Can you work these out from the drawing? Everything is in mm from the part's minimum corner. Give positions to 0.01 mm unless a question says otherwise; leave off trailing zeros. Loops run counter-clockwise (first coordinate to the right, second up) from the corner with the lowest first, then second, coordinate; pieces in that order, holes last. Notation, with made-up numbers: (22, -6.5) -> (81, -6.5) arc R19 ccw to (81, 15.5) -> close; hole circle Ø1 at (54, -25.5). An arc over 180 degrees is marked (long way). Write item = value, one per line. Start each with the question number.
1) I want a section at B-B (z = 0.65). Count the separate pieces of the cut face and the enclosed holes in it, and give its area (3 significant figures).
2) I want a section at C-C (x = 90). List the corners of the cut face in (y, z) for me, and give its area (3 significant figures).
3) I want a section at A-A (y = 15). List the corners of the cut face in (x, z) for me, and give its area (3 significant figures).
4) If we mould it in two halves opening along Z, with no side actions, what happens to the marked faces 1 and 2? For each: +Z half, -Z half, draft (parallel to the pull), parting line (faces both ways), or undercut.
5) I need wall thicknesses on probe 1 along Y at (x, z) = (90, 1.4); probe 2 along X at (y, z) = (6.5, 1.25); probe 3 along X at (y, z) = (34, 0.75). Which ranges of each line are inside material? Lowest first, please. Write a range as from..to.
6) I want a section at D-D (y = 45). List the corners of the cut face in (x, z) for me, and give its area (3 significant figures).
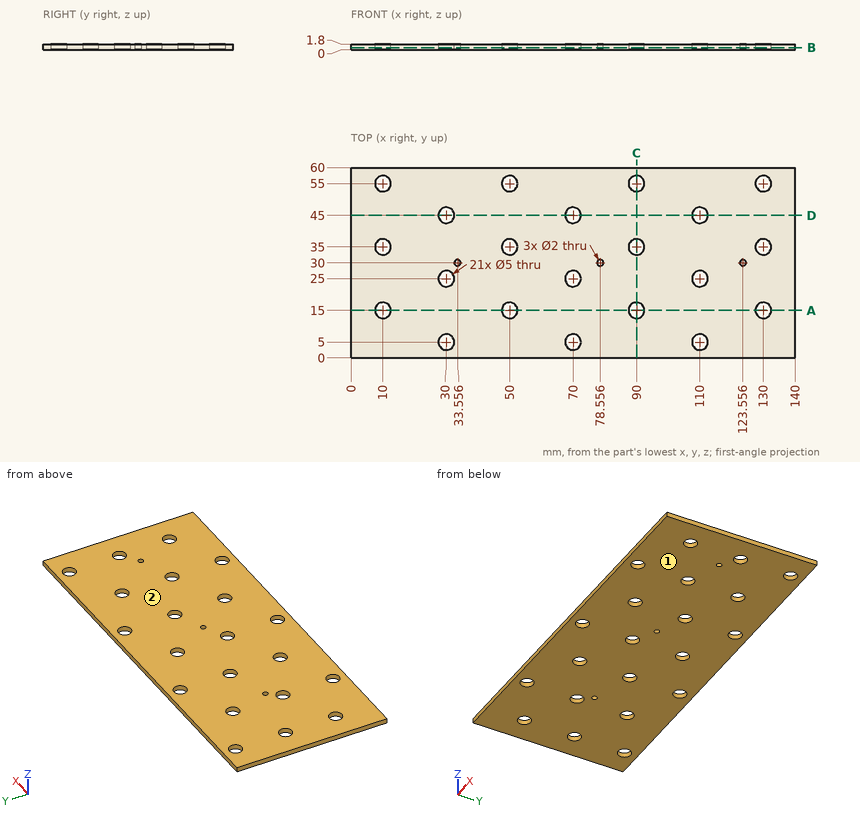
Answer list:
q1.separate_pieces = 1
q1.enclosed_holes = 24
q1.area = 7,980 mm^2
q2.outline = (0, 0) -> (12.5, 0) -> (12.5, 1.8) -> (0, 1.8) -> close; (17.5, 0) -> (32.5, 0) -> (32.5, 1.8) -> (17.5, 1.8) -> close; (37.5, 0) -> (52.5, 0) -> (52.5, 1.8) -> (37.5, 1.8) -> close; (57.5, 0) -> (60, 0) -> (60, 1.8) -> (57.5, 1.8) -> close
q2.area = 81.0 mm^2
q3.outline = (0, 0) -> (7.5, 0) -> (7.5, 1.8) -> (0, 1.8) -> close; (12.5, 0) -> (47.5, 0) -> (47.5, 1.8) -> (12.5, 1.8) -> close; (52.5, 0) -> (87.5, 0) -> (87.5, 1.8) -> (52.5, 1.8) -> close; (92.5, 0) -> (127.5, 0) -> (127.5, 1.8) -> (92.5, 1.8) -> close; (132.5, 0) -> (140, 0) -> (140, 1.8) -> (132.5, 1.8) -> close
q3.area = 216 mm^2
q4.face_1 = -Z half
q4.face_2 = +Z half
q5.probe_1 = 0..12.5, 17.5..32.5, 37.5..52.5, 57.5..60
q5.probe_2 = 0..28, 32..68, 72..108, 112..140
q5.probe_3 = 0..7.71, 12.29..47.71, 52.29..87.71, 92.29..127.71, 132.29..140
q6.outline = (0, 0) -> (27.5, 0) -> (27.5, 1.8) -> (0, 1.8) -> close; (32.5, 0) -> (67.5, 0) -> (67.5, 1.8) -> (32.5, 1.8) -> close; (72.5, 0) -> (107.5, 0) -> (107.5, 1.8) -> (72.5, 1.8) -> close; (112.5, 0) -> (140, 0) -> (140, 1.8) -> (112.5, 1.8) -> close
q6.area = 225 mm^2
